Autodesk Inventor part; units mm, degrees
ref_plane "YZ Plane" through (0, 0, 0) normal (1, 0, 0) x (0, 1, 0)
ref_plane "XZ Plane" through (0, 0, 0) normal (0, 1, 0) x (-1, 0, 0)
ref_plane "XY Plane" through (0, 0, 0) normal (0, 0, 1) x (1, 0, 0)
sketch "Sketch1" plane through (0, 0, 0) normal (0, 1, 0) x (-1, 0, 0)
  line L0 (0, 0) -> (18, 0)
  line L1 (18, 0) -> (18, -20)
  line L2 (18, -20) -> (0, -20)
  line L3 (0, -20) -> (0, 0)
  line L4 (0, 0) -> (0, -5)
  line L5 (0, -5) -> (14, -5)
  line L6 (14, -5) -> (14, -15)
  line L7 (14, -15) -> (0, -15)
  line L8 (0, -15) -> (0, -5)
  dimension "d0" = 18
  dimension "d1" = 20
  dimension "d2" = 5
  dimension "d3" = 14
  dimension "d4" = 10
extrude "Extrusion1" add sketch "Sketch1" along normal blind 8 contours L0 L1 L2 L3 L7 L6 L5
sketch "Sketch2" plane through (0, 0, 0) normal (1, 0, 0) x (0, 0, -1)
  line L0 (20, 8) -> (0, 8)
  line L1 (0, 8) -> (2.5, 8)
  line L2 (2.5, 8) -> (2.5, 4)
  line L3 (2.5, 4) -> (0, 4)
  line L4 (0, 4) -> (0, 8)
  line L5 (20, 0) -> (20, 8)
  line L6 (20, 8) -> (17.5, 8)
  line L7 (17.5, 8) -> (17.5, 4)
  line L8 (17.5, 4) -> (20, 4)
  line L9 (20, 4) -> (20, 8)
  circle A0 centre (2.5, 4) radius 1.5
  circle A1 centre (17.5, 4) radius 1.5
  point P0 (0, 0)
  dimension "d7" = 2.5
  dimension "d8" = 4
  dimension "d9" = 2.5
  dimension "d10" = 4
  dimension "d11" = 3
  dimension "d12" = 3
extrude "Extrusion2" cut sketch "Sketch2" against normal blind 7 contours A1 L8 L7 | L7 L8 A1 | A0 L3 L2 | L2 L3 A0
sketch "Sketch3" plane through (-18, 0, -20) normal (-1, 0, 0) x (0, 0, 1)
  line L0 (0, 0) -> (0, 8)
  line L1 (0, 0) -> (5, 0)
  line L2 (5, 0) -> (5, 4)
  line L3 (5, 4) -> (0, 4)
  line L4 (0, 4) -> (0, 0)
  line L5 (5, 4) -> (15, 4)
  circle A0 centre (5, 4) radius 2
  circle A1 centre (15, 4) radius 2
  point P0 (20, 0)
  dimension "d15" = 5
  dimension "d16" = 4
  dimension "d17" = 10
  dimension "d18" = 4
  dimension "d19" = 4
extrude "Extrusion3" cut sketch "Sketch3" against normal blind 7 contours A1 | A0 L5 L3 | L3 L2 A0 | L2 L5 A0
fillet "Fillet1" radius 2 4 edges at (-9, 8, -20) (-9, 8, 0) (-9, 0, 0) (-9, 0, -20)
properties part number "servo_support_4"
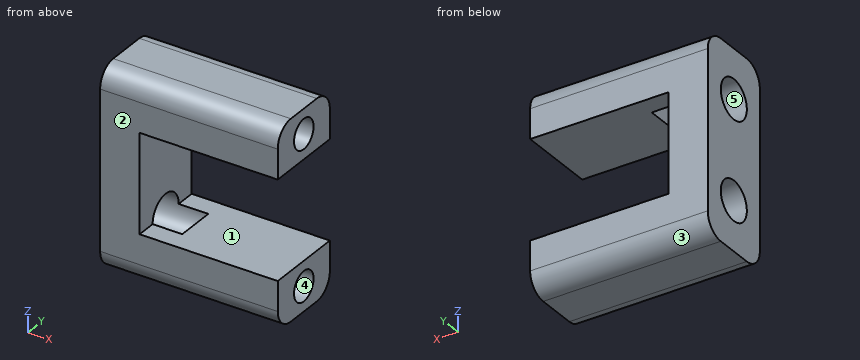
Build history of the part. All positions in model axes, mm. Face numbers are marked on the shaded views. A direction names the side the tool comes from. Coordinates: 2 decimals unless noted, no trailing zeros. Order: outer loops, then holes, each group sorted by start corner. A loop starts at its lowest first (then second) coordinate and runs counter-clockwise, first axis right, second up. Notation, with made-up numbers: M 89,-4 L 128,-4 A18 cw 128,3 Z; hole C 13.5,9.5 d10. An arc over 180 degrees is marked long. One line per question, with ' | ' between items. Start each with the question number.
Q1. Probe L1, parallel to Z at x = -4.5, y = 4; L2, parallel to Z at x = -15, y = 4; L3, parallel to Y at x = -15.75, z = -5. List the from-to ranges inside material, lowest first. Write a range as from..to.
Q2. Saw through at B-B (x = -2.5). List the corners of the cut face in (y, z).
Q3. Saw through at A-A (x = -9). List the corners of the cut face in (y, z), then the cut area to 3 significant figures.
Q4. 3-axis set-ups, long thin cutter, end or side, ignore diameter. For the marked faces 1, 2, 3, 4 and 5: which of +Z, -Z, +X, -X, +Y, -Y reach the whole face in a straight line?
Q5. Saw through at D-D (z = -2.5). List the corners of the cut face in (x, y).
Q6. Saw through at C-C (y = 4). List the corners of the cut face in (x, z).
Q7. Flat gauge pins, fed straight in: pin 1 Ø2.5 at (y, z) = (2, -10.5) entering from +X; pin 2 Ø3.5 at (y, z) = (4, -15) entering from -X. Where does each tip first touch, or does it go through?
Check values:
1) L1: z = -20..-19, -16..-15, -5..-4, -1..0 | L2: z = -20..-17, -13..-7, -3..0 | L3: y = 0..2, 6..8
2) outline: M 0,-18 A2 ccw 2,-20 L 6,-20 A2 ccw 8,-18 L 8,-15 L 0,-15 Z; M 0,-5 L 8,-5 L 8,-2 A2 ccw 6,0 L 2,0 A2 ccw 0,-2 Z; hole C 4,-17.5 d3; hole C 4,-2.5 d3
3) outline: M 0,-18 A2 ccw 2,-20 L 6,-20 A2 ccw 8,-18 L 8,-15 L 0,-15 Z; M 0,-5 L 8,-5 L 8,-2 A2 ccw 6,0 L 2,0 A2 ccw 0,-2 Z | area: 76.6 mm2
4) face 1: +X, +Y, -Y | face 2: +Z, -Z, +X, -X, -Y | face 3: -Z, +X, -X, +Y | face 4: +X | face 5: -X
5) outline: M -18,0 L 0,0 L 0,2.5 L -7,2.5 L -7,5.5 L 0,5.5 L 0,8 L -18,8 Z
6) outline: M -18,-20 L 0,-20 L 0,-19 L -7,-19 L -7,-16 L 0,-16 L 0,-15 L -11,-15 L -11,-17 L -18,-17 Z; M -18,-13 L -14,-13 L -14,-7 L -18,-7 Z; M -18,-3 L -11,-3 L -11,-5 L 0,-5 L 0,-4 L -7,-4 L -7,-1 L 0,-1 L 0,0 L -18,0 Z
7) pin 1: stops at x = -14 | pin 2: stops at x = -11
